Part print with two shaded views. Sizes in mm from the minimum x, y, z corner. Round coordinates to 2 decimals unless told otherwise and drop trailing zeros. Order: outer loops, then holes, each group sorted by start corner. A loop starts at its lowest first (then second) coordinate and runs counter-clockwise, first axis right, second up. Notation, with made-up numbers: M -5.5,51.25 L 19.5,51.25 A15 ccw 19.5,59.25 Z; hole C 44,-33.75 d7. An arc over 180 degrees is marked long. Answer as a JSON object with one key per item and string values.
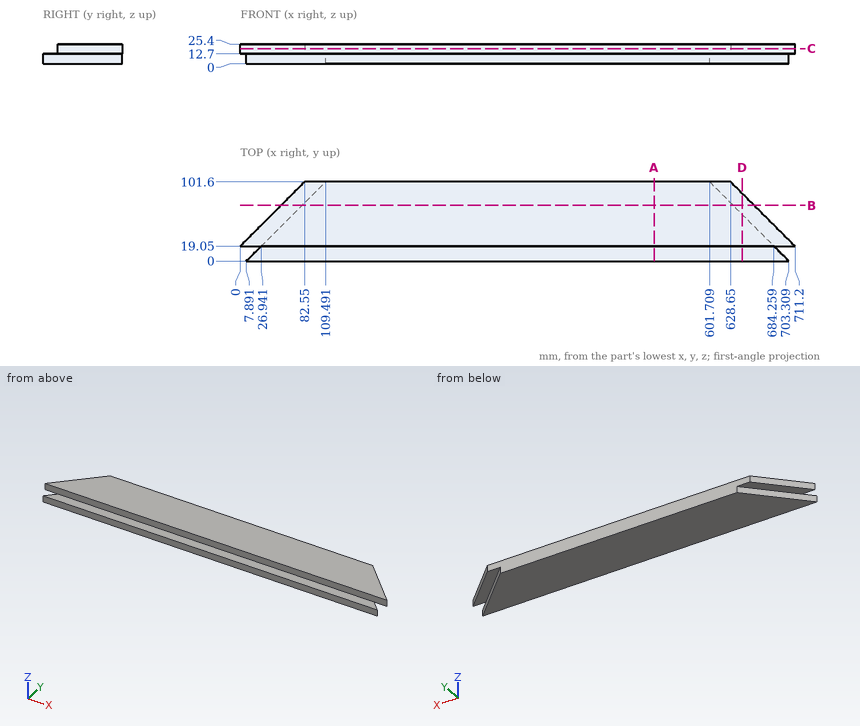
Item 1: Wall check: line 1 along Y through (x, z) = (192.5, 13); line 2 along Y through (x, z) = (70.5, 5.5); line 3 along X through (y, z) = (42, 8.5). Give the ranges that are in metal, low to high. Write a range as [from, to].
Worked answers:
{"line 1": "y = [19.05, 101.6]", "line 2": "y = [0, 62.61]", "line 3": "x = [49.89, 661.31]"}
Item 2: Saw through at C-C on z = 19.5. List the corners of the cut face in (x, y).
Worked answers:
{"outline": "M 0,19.05 L 711.2,19.05 L 628.65,101.6 L 82.55,101.6 Z"}
Item 3: Saw through at D-D on x = 643.5. List the corners of the cut face in (y, z).
Worked answers:
{"outline": "M 0,0 L 59.81,0 L 59.81,12.7 L 86.75,12.7 L 86.75,25.4 L 19.05,25.4 L 19.05,12.7 L 0,12.7 Z"}
Item 4: Drop flat-ended pins along their axis: pin 1 Ø5.5 at (x, y) = (190.5, 8.5) entering from +Z; pin 2 Ø2 at (y, z) = (54, 13) entering from +X; pin 3 Ø10 at (x, z) = (377.5, 20) entering from -Y. Give the stop position or say it passes through.
Worked answers:
{"pin 1": "stops at z = 12.7", "pin 2": "stops at x = 677.25", "pin 3": "stops at y = 19.05"}
Item 5: Saw through at B-B on y = 71.5. List the corners of the cut face in (x, z), and give its area (3 significant figures).
Worked answers:
{"outline": "M 52.45,12.7 L 79.39,12.7 L 79.39,0 L 631.81,0 L 631.81,12.7 L 658.75,12.7 L 658.75,25.4 L 52.45,25.4 Z", "area": "14,700 mm2"}
Item 6: Saw through at A-A on x = 530.5. List the corners of the cut face in (y, z).
Worked answers:
{"outline": "M 0,0 L 101.6,0 L 101.6,25.4 L 19.05,25.4 L 19.05,12.7 L 0,12.7 Z"}
